Check sheet for the modelled part. Datum: model origin and axes. Units: mm. Face numbers are marked on the shaded views. Round coordinates to 2 decimals unless told otherwise and drop trailing zeros. Write each loop counter-clockwise with the first axis right and the second up, starting at its lowest first coordinate (ties: lowest second). Pieces come first, ordered by that corner, then holes. Notation, with made-up numbers: M 49,45.25 L 107,45.25 A17 cw 107,77.25 Z; hole C 44,-12 d3. An arc over 180 degrees is marked long. One line per item, written item: value.
from build123d import *

# Parameters (mm, degrees)
SKETCH087_W   = 83.35
SKETCH087_H   = 40.75
SKETCH087_W_2 = 79.35
SKETCH087_H_2 = 36.75
PAD056_DEPTH  = 0.5
SKETCH088_R   = 1.75
PAD057_DEPTH  = 2
PAD058_DEPTH  = 4


with BuildPart() as part:
    # Sketch087 → Pad056 (new body)
    with BuildSketch(Plane.XY):
        with Locations((2.3, 0)):
            Rectangle(SKETCH087_W, SKETCH087_H)
        with Locations((2.3, 0)):
            Rectangle(SKETCH087_W_2, SKETCH087_H_2, mode=Mode.SUBTRACT)
    extrude(amount=PAD056_DEPTH)

    # Sketch088 (on Face10 of Pad056) → Pad057 (join)
    with BuildSketch(Plane.XY.offset(0.5)):
        with BuildLine():
            Line((-41.625, 22.625), (46.225, 22.625))
            Line((46.225, 22.625), (46.225, 8.656854))
            Line((52.053427, 2.828427), (46.225, 8.656854))
            ThreePointArc((52.053427, -2.828427), (53.225, 0), (52.053427, 2.828427))
            Line((52.053427, -2.828427), (46.225, -8.656854))
            Line((46.225, -8.656854), (46.225, -22.625))
            Line((46.225, -22.625), (-41.625, -22.625))
            Line((-41.625, -22.625), (-41.625, -8.656854))
            Line((-47.453427, -2.828427), (-41.625, -8.656854))
            ThreePointArc((-47.453427, 2.828427), (-48.625, 0), (-47.453427, -2.828427))
            Line((-47.453427, 2.828427), (-41.625, 8.656854))
            Line((-41.625, 8.656854), (-41.625, 22.625))
        make_face()
        with Locations((-44.625, 0)):
            Circle(SKETCH088_R, mode=Mode.SUBTRACT)
        with Locations((49.225, 0)):
            Circle(SKETCH088_R, mode=Mode.SUBTRACT)
    extrude(amount=PAD057_DEPTH)

    # Sketch089 (on Face21 of Pad057) → Pad058 (join)
    with BuildSketch(Plane(origin=(0, 0, 0), x_dir=(1, 0, 0), z_dir=(0, 0, -1))):
        Polygon((-39.375, 20.375), (-39.375, -20.375), (39.375, -20.375), (39.375, -18.375), (-37.375, -18.375), (-37.375, 18.375), (39.375, 18.375), (39.375, 20.375), align=None)
    extrude(amount=PAD058_DEPTH)


with BuildPart() as part_1:
    # Body019 placement: moved
    add(part.part.moved(Location((0, 0, 24.5))))


solid = part_1.part
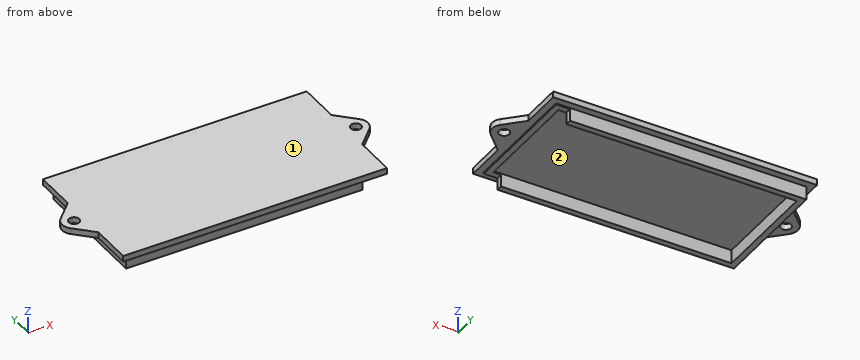
Q1. Sectioned sample at A-A on y = 0. Enter the section's corners in (x, z) (3 decimals).
Completed:
outline: M -48.625,25 L -46.375,25 L -46.375,27 L -48.625,27 Z; M -42.875,25 L -39.375,25 L -39.375,20.5 L -37.375,20.5 L -37.375,25 L 41.975,25 L 41.975,24.5 L 43.975,24.5 L 43.975,25 L 47.475,25 L 47.475,27 L -42.875,27 Z; M 50.975,25 L 53.225,25 L 53.225,27 L 50.975,27 Z
Q2. Sectioned sample at B-B on z = 23. Enter the section's corners in (x, y) (3 decimals).
Completed:
outline: M -39.375,-20.375 L 39.375,-20.375 L 39.375,-18.375 L -37.375,-18.375 L -37.375,18.375 L 39.375,18.375 L 39.375,20.375 L -39.375,20.375 Z
Q3. Sectioned sample at C-C on x = 16. Enter the section's corners in (y, z) (3 decimals).
Completed:
outline: M -22.625,25 L -20.375,25 L -20.375,20.5 L -18.375,20.5 L -18.375,25 L 18.375,25 L 18.375,20.5 L 20.375,20.5 L 20.375,25 L 22.625,25 L 22.625,27 L -22.625,27 Z
Q4. Depth check by flat-ended pin: P1, Ø0.6, axis at y = 2.5, z = 25, coming from the +X side; P2, Ø2, axis at x = 11, z = 22, coming from the +Y side (3 decimals); P3, Ø2, axis at y = -8.5, z = 22, coming from the -X side (3 decimals). Enter the tip coordinate at first touch or a pass-through.
Completed:
P1: x = 52.57
P2: y = 20.375
P3: x = -39.375
Q5. Draft check along Y on the marked faces 1 and 2. Enter one of: pulls with the +Y half, pulls with the -Y half, needs draft (parallel to the pull), parting line crosses it, or undercut.
Completed:
face 1: needs draft
face 2: undercut
Q6. Scan lines: line 1 (Y direction, x = -16.5, z = 22.5) (3 decimals); line 2 (X direction, y = -16, z = 21) (3 decimals); line 3 (Z direction, x = -4, y = 4). Record each from-to range of solid material in increasing order. Write a range as [from, to].
Completed:
line 1: [-20.375, -18.375], [18.375, 20.375]
line 2: [-39.375, -37.375]
line 3: [25, 27]
Q7. Sectioned sample at D-D on y = 7. Enter the section's corners in (x, z) (3 decimals).
Completed:
outline: M -43.282,25 L -39.375,25 L -39.375,20.5 L -37.375,20.5 L -37.375,25 L 41.975,25 L 41.975,24.5 L 43.975,24.5 L 43.975,25 L 47.882,25 L 47.882,27 L -43.282,27 Z
